from build123d import *

# Parameters (mm, degrees)
BOSS_EXTRUDE1_DEPTH = 25.4
SHELL1_T            = -3.175
SKETCH2_R           = 14.3129
CUT_EXTRUDE1_DEPTH  = 456.078410826
SKETCH3_R           = 2.38125
CUT_EXTRUDE2_DEPTH  = 456.078410826
SKETCH4_R           = 2.38125
CUT_EXTRUDE3_DEPTH  = 456.078410826


with BuildPart() as part:
    # Sketch1 → Boss-Extrude1 (new body)
    with BuildSketch(Plane.XY):
        Polygon((0, 0), (203.2, 406.4), (203.2, 292.807746743), (56.796126628, 0), align=None)
    extrude(amount=BOSS_EXTRUDE1_DEPTH)

    # Shell1
    shell1_openings = [part.faces().sort_by_distance(p)[0] for p in [
        (203.2, 349.603873372, 12.7),
        (28.398063314, 0, 12.7),
    ]]
    offset(amount=SHELL1_T, openings=shell1_openings, kind=Kind.INTERSECTION)

    # Sketch2 → Cut-Extrude1 (cut, through all)
    with BuildSketch(Plane.XY.offset(25.4)):
        with Locations((117.298063314, 177.8)):
            Circle(SKETCH2_R)
    extrude(amount=-CUT_EXTRUDE1_DEPTH, mode=Mode.SUBTRACT)

    # Sketch3 → Cut-Extrude2 (cut, through all)
    with BuildSketch(Plane.XY.offset(25.4)):
        with Locations((119.098644425, 203.136098904)):
            Circle(SKETCH3_R)
        with Locations((136.486593771, 194.442124231)):
            Circle(SKETCH3_R)
        with Locations((98.109532857, 161.157875769)):
            Circle(SKETCH3_R)
        with Locations((115.497482204, 152.463901096)):
            Circle(SKETCH3_R)
    extrude(amount=-CUT_EXTRUDE2_DEPTH, mode=Mode.SUBTRACT)

    # Sketch4 → Cut-Extrude3 (cut, through all)
    with BuildSketch(Plane.XY.offset(25.4)):
        with Locations((17.501031657, 6.604)):
            Circle(SKETCH4_R)
        with Locations((45.899094971, 6.604)):
            Circle(SKETCH4_R)
        with Locations((31.661531657, 34.925)):
            Circle(SKETCH4_R)
        with Locations((60.059594971, 34.925)):
            Circle(SKETCH4_R)
        with Locations((166.949905286, 305.501747258)):
            Circle(SKETCH4_R)
        with Locations((178.309130612, 328.22019791)):
            Circle(SKETCH4_R)
        with Locations((192.349905286, 305.501747258)):
            Circle(SKETCH4_R)
    extrude(amount=-CUT_EXTRUDE3_DEPTH, mode=Mode.SUBTRACT)


solid = part.part
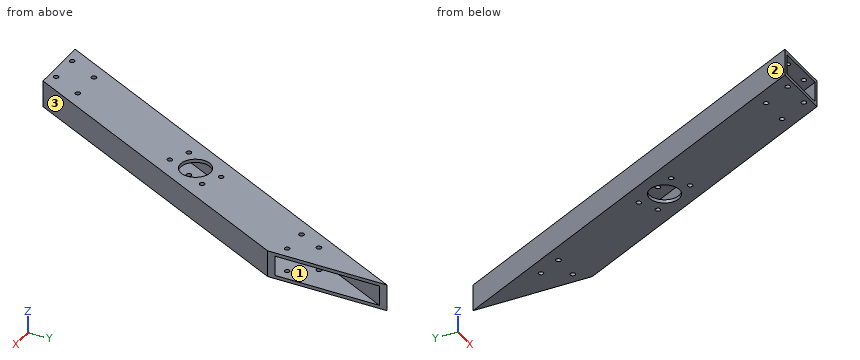
The model under review builds one solid part; all positions refer to its coordinate system, in mm. Face numbers are marked on the shaded views. Give positions to 0.01 mm unless a question says otherwise; leave off trailing zeros. Order: outer loops, then holes, each group sorted by start corner. A loop starts at its lowest first (then second) coordinate and runs counter-clockwise, first axis right, second up. Notation, with made-up numbers: (35.25, 82.5) -> (87.25, 82.5) arc R28 cw to (87.25, 103.5) -> close; hole circle Ø2 at (24, -20). An arc over 180 degrees is marked (long way). Write item = value, one per line. Start each with the question number.
(1) Take a section at C-C (x = 145.5). Write out the cut boundary in (y, z) (3 decimals), plus the area to 3 significant figures.
(2) For L1, parallel to Z at x = 166, y = 285 (3 decimals); L2, parallel to X at y = 90, z = 19.5; L3, parallel to Y at x = 158.5, z = 4.5, list the stretches that pass through material, from the lowest coordinate up. Write a range as from..to.
(3) Take a section at A-A (z = 9.75). Write out the cut boundary in (x, y).
(4) Draft analysis for pull direction X (two halves, no side actions). For the marked faces 1, 2 and 3, state which applies: +X half, -X half, draft (parallel to the pull), parting line (faces both ways), or undercut.
(5) For pin 1 Ø3 at (x, z) = (95.5, 19) entering from +Y; pin 2 Ø12 at (y, z) = (49.5, 5.5) entering from -X; pin 3 Ø3 at (x, y) = (115.5, 152.46) entering from +Z (3 decimals); pin 4 Ø3 at (x, z) = (96.5, 7) entering from -Y, all flat-tipped, find the tip position at first contact; note any pin that passes through.
(6) Take a section at B-B (y = 177.8). Write out the cut boundary in (x, z) (3 decimals).
(7) Take a section at D-D (y = 43.5). Write out the cut boundary in (x, z) (3 decimals), plus the area to 3 significant figures.
Returned:
q1.outline = (177.408, 0) -> (291, 0) -> (291, 25.4) -> (177.408, 25.4) -> close; hole (184.507, 3.175) -> (283.9, 3.175) -> (283.9, 22.225) -> (184.507, 22.225) -> close
q1.area = 992 mm²
q2.L1 = 0..3.175, 22.225..25.4
q2.L2 = 45..48.55, 98.25..101.8
q2.L3 = 203.41..210.51, 309.9..317
q3.outline = (0, 0) -> (3.55, 0) -> (203.2, 399.3) -> (203.2, 406.4) -> close; (53.25, 0) -> (56.8, 0) -> (203.2, 292.81) -> (203.2, 299.91) -> close
q4.face_1 = undercut
q4.face_2 = -X half
q4.face_3 = +X half
q5.pin_1 = 194
q5.pin_2 = 21.75
q5.pin_3 = through
q5.pin_4 = 76.41
q6.outline = (88.9, 0) -> (102.985, 0) -> (102.985, 3.175) -> (92.45, 3.175) -> (92.45, 22.225) -> (102.985, 22.225) -> (102.985, 25.4) -> (88.9, 25.4) -> close; (131.611, 0) -> (145.696, 0) -> (145.696, 25.4) -> (131.611, 25.4) -> (131.611, 22.225) -> (142.146, 22.225) -> (142.146, 3.175) -> (131.611, 3.175) -> close
q7.outline = (21.75, 0) -> (78.546, 0) -> (78.546, 25.4) -> (21.75, 25.4) -> close; hole (25.3, 3.175) -> (74.996, 3.175) -> (74.996, 22.225) -> (25.3, 22.225) -> close
q7.area = 496 mm²
